Read the model definition and answer for the solid it produces. Units are mm, in the model's axes. Give positions to 0.01 mm unless a question says otherwise; leave off trailing zeros. Order: outer loops, then holes, each group sorted by start corner. A loop starts at its lowest first (then second) coordinate and runs counter-clockwise, first axis right, second up. Notation, with made-up numbers: (65, 75) -> (119, 75) arc R21 cw to (119, 107) -> close; hole circle Ø2 at (-39, 33). An arc over 180 degrees is marked (long way). One line per item, written item: value. Start each with the question number.
Autodesk Inventor part; units mm, degrees
ref_plane "YZ Plane" through (0, 0, 0) normal (1, 0, 0) x (0, 1, 0)
ref_plane "XZ Plane" through (0, 0, 0) normal (0, 1, 0) x (-1, 0, 0)
ref_plane "XY Plane" through (0, 0, 0) normal (0, 0, 1) x (1, 0, 0)
sketch "Sketch1" plane through (0, 0, 0) normal (0, 0, 1) x (1, 0, 0)
  line L0 (-26, 13) -> (26, 13)
  line L1 (26, -13) -> (-26, -13)
  line L2 (-26, 13) -> (26, -13) construction
  line L3 (26, 13) -> (-26, -13) construction
  line L4 (-54.6, 15.6) -> (54.6, 15.6)
  line L5 (54.6, 15.6) -> (54.6, -15.6)
  line L6 (54.6, -15.6) -> (-54.6, -15.6)
  line L7 (-54.6, -15.6) -> (-54.6, 15.6)
  line L8 (-54.6, 15.6) -> (54.6, -15.6) construction
  line L9 (54.6, 15.6) -> (-54.6, -15.6) construction
  line L10 (-26, 1.3) -> (-35.75, 1.3)
  line L11 (-35.75, 1.3) -> (-35.75, -1.3)
  line L12 (-35.75, -1.3) -> (-26, -1.3)
  line L13 (26, 1.3) -> (35.75, 1.3)
  line L14 (35.75, 1.3) -> (35.75, -1.3)
  line L15 (35.75, -1.3) -> (26, -1.3)
  line L16 (-26, 1.3) -> (-26, 13)
  line L17 (-26, -13) -> (-26, -1.3)
  line L18 (26, -1.3) -> (26, -13)
  line L19 (26, 1.3) -> (26, 13)
  point P0 (0, 0)
  point P1 (-35.75, 0)
  point P2 (0, 0)
  dimension "CInt" = 52
  dimension "LInt" = 26
  dimension "Cext" = 109.2
  dimension "Lext" = 31.2
  dimension "Cpeq" = 9.75
  dimension "Lpeq" = 2.6
  dimension "d10" = 9.75
  dimension "d11" = 2.6
extrude "Extrusion1" add sketch "Sketch1" along normal mid plane 6.5
sketch "Sketch8" plane through (0, 0, 3.25) normal (0, 0, 1) x (1, 0, 0)
  point P0 (0, 0)
hole "Hole1" at (-32.5, 6.5, 3.25) direction (0, 0, -1) diameter 6.5 end through all
pattern_linear "Rectangular Pattern1" count 2 spacing 13 along (0, -1, 0) of "Hole1"
hole "Hole2" at (32.5, 6.5, 3.25) direction (0, 0, -1) diameter 6.5 end through all
pattern_linear "Rectangular Pattern2" count 2 spacing 13 along (0, -1, 0) of "Hole2"
properties part number "Cou-2"
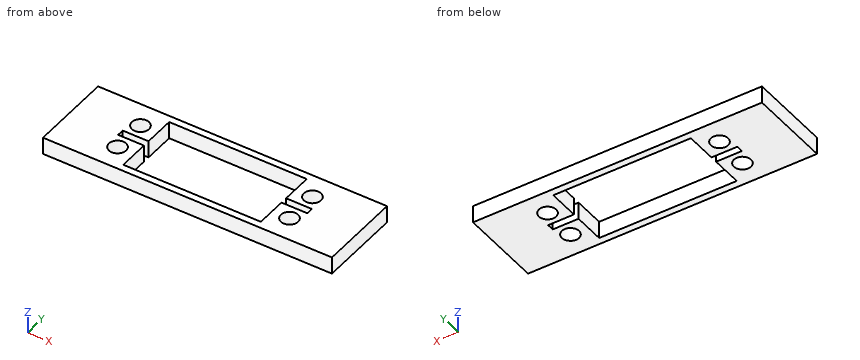
Item 1: Find section A-A on x = 9. Write down the section's boundary in (y, z).
Item 2: Find section B-B on z = -1.75. Write down the section's boundary in (x, y), then the cut area to 3 significant figures.
Item 3: Find section D-D on y = -12. Write down the section's boundary in (x, z).
Item 4: Find the intervals of material crossed by line 1 (X direction, y = 6.5, z = -0.75); line 2 (Y direction, x = -32.5, z = 1.25); line 3 (Y direction, x = 23, z = 0.25), in increasing order. Write a range as from..to.
Item 5: Find section C-C on x = -32.5. Write down the section's boundary in (y, z).
Checks:
1. outline: (-15.6, -3.25) -> (-13, -3.25) -> (-13, 3.25) -> (-15.6, 3.25) -> close; (13, -3.25) -> (15.6, -3.25) -> (15.6, 3.25) -> (13, 3.25) -> close
2. outline: (-54.6, -15.6) -> (54.6, -15.6) -> (54.6, 15.6) -> (-54.6, 15.6) -> close; hole circle Ø6.5 at (-32.5, -6.5); hole (-35.75, -1.3) -> (-26, -1.3) -> (-26, -13) -> (26, -13) -> (26, -1.3) -> (35.75, -1.3) -> (35.75, 1.3) -> (26, 1.3) -> (26, 13) -> (-26, 13) -> (-26, 1.3) -> (-35.75, 1.3) -> close; hole circle Ø6.5 at (-32.5, 6.5); hole circle Ø6.5 at (32.5, -6.5); hole circle Ø6.5 at (32.5, 6.5)
2. area: 1,870 mm2
3. outline: (-54.6, -3.25) -> (-26, -3.25) -> (-26, 3.25) -> (-54.6, 3.25) -> close; (26, -3.25) -> (54.6, -3.25) -> (54.6, 3.25) -> (26, 3.25) -> close
4. line 1: -54.6..-35.75, -29.25..-26, 26..29.25, 35.75..54.6
4. line 2: -15.6..-9.75, -3.25..-1.3, 1.3..3.25, 9.75..15.6
4. line 3: -15.6..-13, 13..15.6
5. outline: (-15.6, -3.25) -> (-9.75, -3.25) -> (-9.75, 3.25) -> (-15.6, 3.25) -> close; (-3.25, -3.25) -> (-1.3, -3.25) -> (-1.3, 3.25) -> (-3.25, 3.25) -> close; (1.3, -3.25) -> (3.25, -3.25) -> (3.25, 3.25) -> (1.3, 3.25) -> close; (9.75, -3.25) -> (15.6, -3.25) -> (15.6, 3.25) -> (9.75, 3.25) -> close
